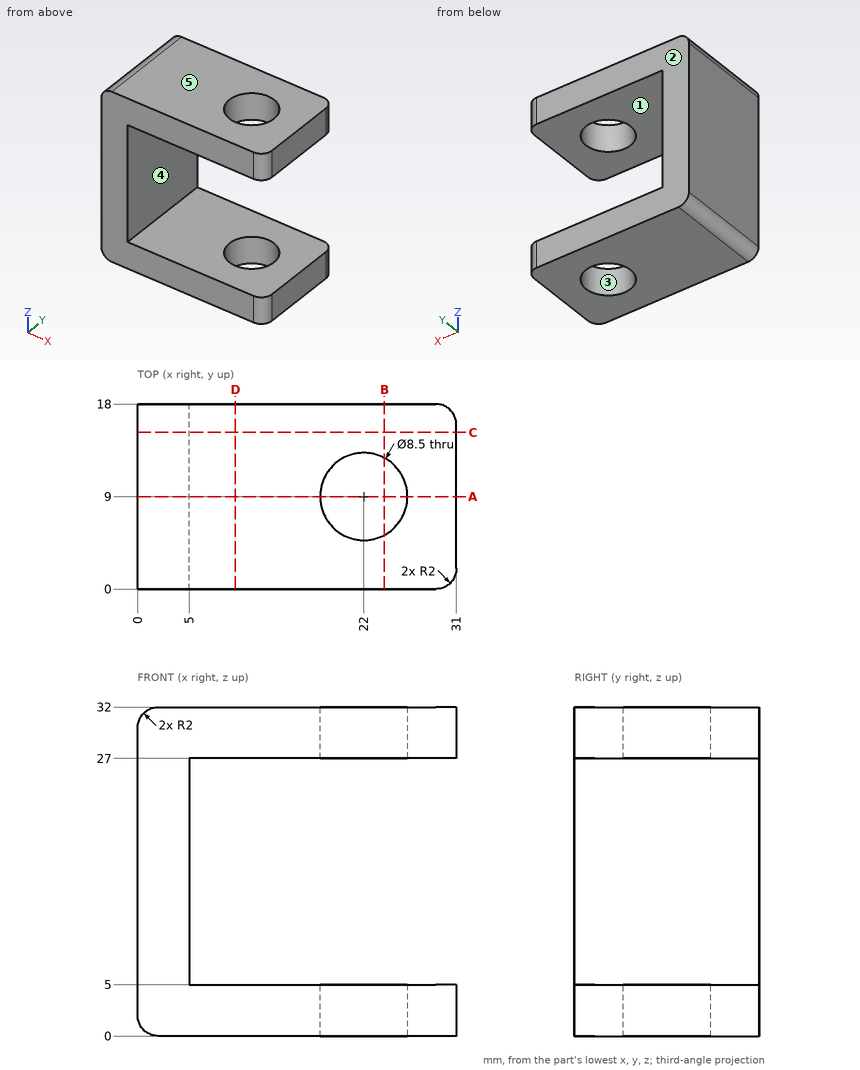
The figure shows three views and two pictorial views of one solid part (mm, origin at its lowest corner). Answer the questions. A direction names the side the tool comes from. Give positions to 0.01 mm unless a question says otherwise; leave off trailing zeros. Write each loop counter-clockwise with the first axis right and the second up, starting at its lowest first coordinate (ties: lowest second). Pieces come first, ordered by that corner, then holes. Notation, with made-up numbers: (-3, 53) - (10, 53) arc R12 ccw to (10, 75) - close; hole circle Ø10 at (27.5, -23). An arc over 180 degrees is marked (long way). Use one line per item in the form item = value.
1. Each of these flat-tipped pins is pushed along its axis until it touches: pin 1 Ø1.5 at (x, y) = (24.5, 10.5) entering from -Z; pin 2 Ø5.5 at (x, y) = (19, 10) entering from +Z; pin 3 Ø4 at (y, z) = (12, 9.5) entering from +X. Where does it stop, or does it pass through?
Filled in:
pin_1 = through
pin_2 = 32
pin_3 = 5
2. Determine the mould class of the marked faces 3, 4 and 5 for opening direction Z: released by +Z, released by -Z, zero draft, split by the parting line, or undercut.
Filled in:
face_3 = zero draft
face_4 = undercut
face_5 = released by +Z
3. A cutting plane is placed at B-B (x = 24). Write down the section's boundary in (y, z), and give its area (3 significant figures).
Filled in:
outline = (0, 0) - (5.25, 0) - (5.25, 5) - (0, 5) - close; (0, 27) - (5.25, 27) - (5.25, 32) - (0, 32) - close; (12.75, 0) - (18, 0) - (18, 5) - (12.75, 5) - close; (12.75, 27) - (18, 27) - (18, 32) - (12.75, 32) - close
area = 105 mm^2
4. A cutting plane is placed at C-C (y = 15.25). Write down the section's boundary in (x, z).
Filled in:
outline = (0, 2) arc R2 ccw to (2, 0) - (31, 0) - (31, 5) - (5, 5) - (5, 27) - (31, 27) - (31, 32) - (2, 32) arc R2 ccw to (0, 30) - close
5. Consider L1, parallel to Z at x = 13.5, y = 4.5; L2, parallel to Y at x = 22, z = 2; L3, parallel to X at y = 3, z = 12. Determine where each line is inside the solid, lowest interval first.
Filled in:
L1 = 0 to 5, 27 to 32
L2 = 0 to 4.75, 13.25 to 18
L3 = 0 to 5
6. For the marked faces 1 and 2, determine the directions among +Z, -Z, +X, -X, +Y, -Y from which every point of the face is accessible in a straight line to the end or side of a thin tool.
Filled in:
face_1 = +X, +Y, -Y
face_2 = +Z, -Z, +X, -X, +Y
7. A cutting plane is placed at A-A (y = 9). Write down the section's boundary in (x, z).
Filled in:
outline = (0, 2) arc R2 ccw to (2, 0) - (17.75, 0) - (17.75, 5) - (5, 5) - (5, 27) - (17.75, 27) - (17.75, 32) - (2, 32) arc R2 ccw to (0, 30) - close; (26.25, 0) - (31, 0) - (31, 5) - (26.25, 5) - close; (26.25, 27) - (31, 27) - (31, 32) - (26.25, 32) - close
8. A cutting plane is placed at D-D (x = 9.5). Write down the section's boundary in (y, z).
Filled in:
outline = (0, 0) - (18, 0) - (18, 5) - (0, 5) - close; (0, 27) - (18, 27) - (18, 32) - (0, 32) - close
